from build123d import *

# Parameters (mm, degrees)
F0_R     = 58.262623
F1_DEPTH = 34.544
F2_DEPTH = 63.754


with BuildPart() as f1:
    # F0 (on Front) → F1 (new body)
    with BuildSketch(Plane.XZ):
        Circle(F0_R)
        with BuildLine():
            ThreePointArc((25.805285, 27.944596), (34.845149, 15.252174), (38.036998, 0))
            ThreePointArc((38.036998, 0), (35.17286, -14.480438), (27.01178, -26.780159))
            ThreePointArc((27.01178, -26.780159), (14.631752, -35.110184), (0, -38.036998))
            ThreePointArc((0, -38.036998), (-15.583326, -34.698316), (-28.431013, -25.268374))
            ThreePointArc((-28.431013, -25.268374), (-35.55449, -13.516339), (-38.036998, 0))
            ThreePointArc((-38.036998, 0), (-35.902258, 12.56348), (-29.737655, 23.716767))
            ThreePointArc((-29.737655, 23.716767), (-16.503008, 34.270452), (0, 38.036998))
            ThreePointArc((0, 38.036998), (13.854325, 35.424156), (25.805285, 27.944596))
        make_face(mode=Mode.SUBTRACT)
    extrude(amount=F1_DEPTH)

    # F0 (on Front) → F2 (join)
    with BuildSketch(Plane.XZ):
        Circle(F0_R)
        with BuildLine():
            ThreePointArc((25.805285, 27.944596), (34.845149, 15.252174), (38.036998, 0))
            ThreePointArc((38.036998, 0), (35.17286, -14.480438), (27.01178, -26.780159))
            ThreePointArc((27.01178, -26.780159), (14.631752, -35.110184), (0, -38.036998))
            ThreePointArc((0, -38.036998), (-15.583326, -34.698316), (-28.431013, -25.268374))
            ThreePointArc((-28.431013, -25.268374), (-35.55449, -13.516339), (-38.036998, 0))
            ThreePointArc((-38.036998, 0), (-35.902258, 12.56348), (-29.737655, 23.716767))
            ThreePointArc((-29.737655, 23.716767), (-16.503008, 34.270452), (0, 38.036998))
            ThreePointArc((0, 38.036998), (13.854325, 35.424156), (25.805285, 27.944596))
        make_face(mode=Mode.SUBTRACT)
    extrude(amount=F2_DEPTH)


solid = f1.part
Could you check a few things on this model? Use its own coordinates, in mm. Coordinates: 2 decimals unless noted, no trailing zeros. Order: outer loops, then holes, each group sorted by start corner. A loop starts at its lowest first (then second) coordinate and runs counter-clockwise, first axis right, second up. Notation, with made-up numbers: (77, -6) - (110, -6) arc R29 cw to (110, 24) - close; hole circle Ø9 at (-2, -0.5). An arc over 180 degrees is marked (long way). Answer in a Markdown table with one row per item. Add a question column.
(1) I need wall thicknesses on L1, parallel to Z at x = 7, y = -50; L2, parallel to X at y = -60, z = 9.5; L3, parallel to X at y = -18, z = -22.5. Which ranges of each line are inside material? Lowest first, please.
(2) If we section it at D-D, the plane x = 45.5: Please give me the cut outline in (y, z).
(3) If we section it at B-B, the plane z = 19.5: Please give me the cut outline in (x, y).
(4) If we section it at C-C, the plane y = -21.5: Please give me the cut outline in (x, z).
(5) Will these pins go through, and if not, where does the flat tip stop? pin 1 (1.5 mm diameter, centred on y = -47.5, z = 26, fed in from +X); pin 2 (3 mm diameter, centred on x = 24, y = -20.5, fed in from -Z); pin 3 (12 mm diameter, centred on x = -3, y = -42, fed in from +Z).
(6) If we section it at A-A, the plane x = 5: Please give me the cut outline in (y, z), then the cut area to 3 significant figures.
Results are:
| question | item | result |
|---|---|---|
| 1 | L1 | z = -57.84 to -37.39, 37.39 to 57.84 |
| 1 | L2 | x = -57.48 to -36.83, 36.83 to 57.48 |
| 1 | L3 | x = -53.74 to -30.67, 30.67 to 53.74 |
| 2 | outline | (-63.75, -36.39) - (0, -36.39) - (0, 36.39) - (-63.75, 36.39) - close |
| 3 | outline | (-54.9, -63.75) - (-32.66, -63.75) - (-32.66, 0) - (-54.9, 0) - close; (32.66, -63.75) - (54.9, -63.75) - (54.9, 0) - (32.66, 0) - close |
| 4 | outline | circle Ø116.53 at (0, 0); hole (-38.04, 0) arc R38.04 ccw to (-28.43, -25.27) arc R38.04 ccw to (0, -38.04) arc R38.04 ccw to (27.01, -26.78) arc R38.04 ccw to (38.04, 0) arc R38.04 ccw to (25.81, 27.94) arc R38.04 ccw to (0, 38.04) arc R38.04 ccw to (-29.74, 23.72) arc R38.04 ccw to start |
| 5 | pin 1 | stops at x = 52.51 |
| 5 | pin 2 | stops at z = -53.74 |
| 5 | pin 3 | stops at z = 58.26 |
| 6 | outline | (-63.75, -58.05) - (0, -58.05) - (0, -37.71) - (-63.75, -37.71) - close; (-63.75, 37.71) - (0, 37.71) - (0, 58.05) - (-63.75, 58.05) - close |
| 6 | area | 2,590 mm2 |
